```python
from build123d import *

# Parameters (mm, degrees)
RESSALTO_EXTRUS_O1_DEPTH = 10
ESBO_O3_R                = 1.7
CORTE_EXTRUS_O1_DEPTH    = 33.009811874
CORTE_EXTRUS_O3_START    = -11.4
ESBO_O3_4_R              = 1.7
CORTE_EXTRUS_O3_DEPTH    = 3


with BuildPart() as part:
    # Esboço2 → Ressalto-extrusão1 (new body)
    with BuildSketch(Plane.XY):
        Polygon((-49.807026949, 9.042797905), (-32.734806181, 38.612751673), (-20.264040367, 31.412751673), (-37.336261135, 1.842797905), align=None)
    extrude(amount=RESSALTO_EXTRUS_O1_DEPTH)

    # Esboço3 → Corte-extrusão1 (cut, through all)
    with BuildSketch(Plane(origin=(-41.270916565, 23.827774789, 0), x_dir=(0, 0, 1), z_dir=(-0.8660254037844386, 0.5000000000000003, 0))):
        with Locations(Location((5, 0, 0), (0, 0, 270))):
            Circle(ESBO_O3_R)
    extrude(amount=-CORTE_EXTRUS_O1_DEPTH, mode=Mode.SUBTRACT)

    # Esboço3<4> → Corte-extrusão3 (cut)
    with BuildSketch(Plane(origin=(-41.270916565, 23.827774789, 0), x_dir=(0, 0, 1), z_dir=(-0.8660254037844386, 0.5000000000000003, 0)).offset(CORTE_EXTRUS_O3_START)):
        Polygon((4.988193566, 3.524626071), (1.988193566, 1.792575264), (1.988193566, -1.671526352), (4.988193566, -3.403577159), (7.988193566, -1.671526352), (7.988193566, 1.792575264), align=None)
        with Locations(Location((5, 0, 0), (0, 0, 270))):
            Circle(ESBO_O3_4_R, mode=Mode.SUBTRACT)
    extrude(amount=-CORTE_EXTRUS_O3_DEPTH, mode=Mode.SUBTRACT)


solid = part.part
```
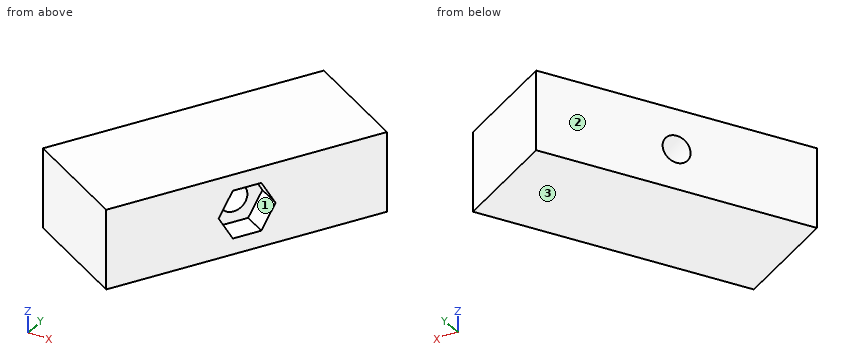
Design review of the part built by this model. Coordinates are the model's own, in mm. Face numbers are marked on the shaded views. Coordinates: 2 decimals unless noted, no trailing zeros. Order: outer loops, then holes, each group sorted by start corner. A loop starts at its lowest first (then second) coordinate and runs counter-clockwise, first axis right, second up. Notation, with made-up numbers: (8.25, 16.25) -> (20.25, 16.25) arc R13 cw to (20.25, 26.25) -> close; hole circle Ø3 at (63.5, 3.25). An arc over 180 degrees is marked (long way). One line per item, written item: value. Start each with the question number.
Q1. Insertion check: pin 1 Ø1 at (y, z) = (12, 2) entering from -X; pin 2 Ø1.5 at (y, z) = (31.5, 7.5) entering from -X; pin 3 Ø4 at (x, z) = (-44.5, 8.5) entering from -Y. Each pin has a flat end and moves straight along its axis. Give the tip position at first contact, or say it passes through.
Q2. Take a section at C-C, the plane y = 33. State the section outline as (x, z) points.
Q3. Take a section at A-A, the plane x = -29.25. State the section outline as (y, z) points, then the cut area to 3 significant figures.
Q4. Take a section at D-D, the plane z = 2.75. State the section outline as (x, y) points.
Q5. For probe 1 along Z at (x, y) = (-41, 23); probe 2 along X at (y, z) = (19.5, 2.5); probe 3 along Y at (x, z) = (-37.25, 4), list the stretches that pass through material, from the lowest coordinate up.
Q6. Mouldability with a two-part tool opening along Z and no side actions: class the marked faces 1, 2 and 3 as pulls with the +Z half, pulls with the -Z half, needs draft (parallel to the pull), parting line crosses it, or undercut.
Q7. Take a section at B-B, the plane z = 9.25. State the section outline as (x, y) points.
Values follow:
1. pin 1: stops at x = -48.39
1. pin 2: stops at x = -37.27
1. pin 3: stops at y = 4.82
2. outline: (-35.98, 0) -> (-23.01, 0) -> (-23.01, 10) -> (-35.98, 10) -> close
3. outline: (15.85, 0) -> (36.6, 0) -> (36.6, 10) -> (15.85, 10) -> (15.85, 7.99) -> (18.96, 7.99) -> (20.96, 4.99) -> (18.96, 1.99) -> (15.85, 1.99) -> close
3. area: 183 mm2
4. outline: (-49.81, 9.04) -> (-37.34, 1.84) -> (-29.86, 14.8) -> (-32.45, 16.3) -> (-30.28, 20.06) -> (-27.68, 18.56) -> (-20.26, 31.41) -> (-32.73, 38.61) -> close
5. probe 1: z = 0 to 3.4, 6.6 to 10
5. probe 2: x = -43.77 to -30.61, -29.6 to -27.14
5. probe 3: y = 1.99 to 19.92, 23.09 to 30.79
6. face 1: undercut
6. face 2: needs draft
6. face 3: pulls with the -Z half
7. outline: (-49.81, 9.04) -> (-37.34, 1.84) -> (-20.26, 31.41) -> (-32.73, 38.61) -> close
